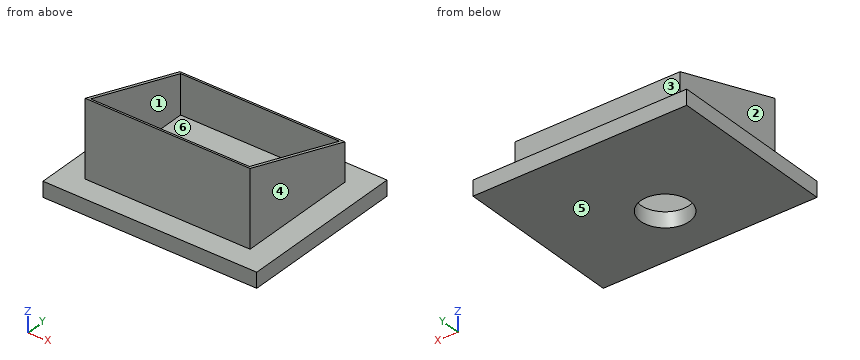
```python
from build123d import *

# Parameters (mm, degrees)
SKETCH2_W           = 700
SKETCH2_H           = 550
BOSS_EXTRUDE1_DEPTH = 50
SKETCH3_W           = 540
SKETCH3_H           = 400
SKETCH3_W_2         = 520
SKETCH3_H_2         = 380
EXTRUDE_THIN1_DEPTH = 250
CUT_EXTRUDE1_DEPTH  = 621
SKETCH7_R           = 80
CUT_EXTRUDE2_DEPTH  = 51


with BuildPart() as part:
    # Sketch2 → Boss-Extrude1 (new body)
    with BuildSketch(Plane.XY):
        Rectangle(SKETCH2_W, SKETCH2_H)
    extrude(amount=BOSS_EXTRUDE1_DEPTH)

    # Sketch3 → Extrude-Thin1 (add)
    with BuildSketch(Plane.XY.offset(50)):
        Rectangle(SKETCH3_W, SKETCH3_H)
        Rectangle(SKETCH3_W_2, SKETCH3_H_2, mode=Mode.SUBTRACT)
    extrude(amount=EXTRUDE_THIN1_DEPTH)

    # Sketch4 → Cut-Extrude1 (cut, through all)
    with BuildSketch(Plane.ZY.offset(270)):
        Polygon((175, 200), (300, -200), (300, 200), align=None)
    extrude(amount=-CUT_EXTRUDE1_DEPTH, mode=Mode.SUBTRACT)

    # Sketch7 → Cut-Extrude2 (cut, through all)
    with BuildSketch(Plane.XY.offset(50)):
        with Locations((0, -85)):
            Circle(SKETCH7_R)
    extrude(amount=-CUT_EXTRUDE2_DEPTH, mode=Mode.SUBTRACT)


solid = part.part
```
For this review, take the finished solid that the model builds, in its own axes (mm). Face numbers are marked on the shaded views. A direction names the side the tool comes from. Coordinates: 2 decimals unless noted, no trailing zeros. Order: outer loops, then holes, each group sorted by start corner. A loop starts at its lowest first (then second) coordinate and runs counter-clockwise, first axis right, second up. Notation, with made-up numbers: (-8.75, -7.5) - (46.25, -7.5) arc R15 ccw to (46.25, 13.5) - close; hole circle Ø6 at (48.25, -29). An arc over 180 degrees is marked (long way). Answer as a JSON object with one key per item and string values. Group by question number.
1. For the marked faces 1, 2 and 3, list the 3-axis set-ups (+Z, -Z, +X, -X, +Y, -Y) from which the entire face can be reached by the end or side of a thin tool; tool diameter is ignored.
2. For probe 1 along X at (y, z) = (124, 140); probe 2 along Y at (x, z) = (0, 10); probe 3 along Z at (x, y) = (-180, 74), list the stretches that pass through material, from the lowest coordinate up.
3. The part is to be moulded in two halves that separate along X. For the marked faces 4, 5 and 6, say which applies: pulls with the +X half, pulls with the -X half, needs draft (parallel to the pull), parting line crosses it, or undercut.
4. Clearance check with flat-ended pins moving along their axes: P1, Ø1, axis at x = -190.5, y = 86.5, coming from the +Z side; P2, Ø6, axis at x = 246.5, z = 116.5, coming from the +Y side; P3, Ø6, axis at y = 6, z = 216, coming from the -X side. State where each tip first meets the part, or that it passes through.
5. We need section C-C on y = -85. State the section outline as (x, z) points.
6. We need section A-A on x = 0. State the section outline as (y, z) points (3 decimals).
7. We need section D-D on x = 216. State the section outline as (y, z) points (3 decimals), then the cut area to 4 significant figures.
8. We need section B-B on z = 81.5. State the section outline as (x, y) points, then the cut area to 3 significant figures.
Final values:
{
 "1": {"face 1": "+Z", "face 2": "+Z, -X, +Y, -Y", "face 3": "+Z, +X, -X, +Y"},
 "2": {"probe 1": "-270 to -260, 260 to 270", "probe 2": "-275 to -165, -5 to 275", "probe 3": "0 to 50"},
 "3": {"face 4": "pulls with the +X half", "face 5": "needs draft", "face 6": "undercut"},
 "4": {"P1": "z = 50", "P2": "y = 200", "P3": "x = -270"},
 "5": {"outline": "(-350, 0) - (-80, 0) - (-80, 50) - (-260, 50) - (-260, 264.06) - (-270, 264.06) - (-270, 50) - (-350, 50) - close; (80, 0) - (350, 0) - (350, 50) - (270, 50) - (270, 264.06) - (260, 264.06) - (260, 50) - (80, 50) - close"},
 "6": {"outline": "(-275, 0) - (-165, 0) - (-165, 50) - (-190, 50) - (-190, 296.875) - (-200, 300) - (-200, 50) - (-275, 50) - close; (-5, 0) - (275, 0) - (275, 50) - (200, 50) - (200, 175) - (190, 178.125) - (190, 50) - (-5, 50) - close"},
 "7": {"outline": "(-275, 0) - (275, 0) - (275, 50) - (200, 50) - (200, 175) - (190, 178.125) - (190, 50) - (-190, 50) - (-190, 296.875) - (-200, 300) - (-200, 50) - (-275, 50) - close", "area": "31,250 mm²"},
 "8": {"outline": "(-270, -200) - (270, -200) - (270, 200) - (-270, 200) - close; hole (-260, -190) - (260, -190) - (260, 190) - (-260, 190) - close", "area": "18,400 mm²"}
}
